Design review of the part built by this model. Coordinates are the model's own, in mm. A direction names the side the tool comes from. Give positions to 0.01 mm unless a question says otherwise; leave off trailing zeros. Write each loop counter-clockwise with the first axis right and the second up, starting at its lowest first coordinate (ties: lowest second). Pieces come first, ordered by that corner, then holes. Notation, with made-up numbers: (-7.5, 32) -> (17.5, 32) arc R24 cw to (17.5, 66) -> close; hole circle Ø7 at (35.25, 50.5). An arc over 180 degrees is marked (long way). Answer as a JSON object with one key per item and string values.
```python
from build123d import *

# Parameters (mm, degrees)
F1_DEPTH = 233
F2_R     = 8.5
F3_DEPTH = 20
F4_R     = 12.5
F5_DEPTH = 15
F7_DEPTH = 15


with BuildPart() as f1:
    # F0 (on Top) → F1 (new body)
    with BuildSketch(Plane.XY):
        Polygon((5, 8.660254), (-5, 8.660254), (-10, 0), (-5, -8.660254), (5, -8.660254), (10, 0), align=None)
    extrude(amount=F1_DEPTH)

    # F2 (on face) → F3 (join)
    with BuildSketch(Plane.XY.offset(233)):
        Circle(F2_R)
    extrude(amount=F3_DEPTH)

    # F4 (on face) → F5 (join)
    with BuildSketch(Plane(origin=(0, 0, 0), x_dir=(1, 0, 0), z_dir=(0, 0, -1))):
        Circle(F4_R)
        Polygon((5, -8.660254), (-5, -8.660254), (-10, 0), (-5, 8.660254), (5, 8.660254), (10, 0), align=None, mode=Mode.SUBTRACT)
        Polygon((-10, 0), (-5, -8.660254), (5, -8.660254), (10, 0), (5, 8.660254), (-5, 8.660254), align=None)
    extrude(amount=F5_DEPTH)

    # F6 (on face) → F7 (join)
    with BuildSketch(Plane(origin=(0, 0, -15), x_dir=(1, 0, 0), z_dir=(0, 0, -1))):
        Polygon((4.953786, -8.686772), (9.999858, -0.053281), (5.046072, 8.633491), (-4.953786, 8.686772), (-9.999858, 0.053281), (-5.046072, -8.633491), align=None)
    extrude(amount=F7_DEPTH)


solid = f1.part
```
(1) For line 1 along Z through (x, y) = (5.5, -8.5); line 2 along Y through (x, z) = (1, 92.5); line 3 along Y through (x, z) = (-0.75, 238), list the stretches that pass through material, from the lowest coordinate up.
Here are the results:
{"line 1": "z = -15 to 0", "line 2": "y = -8.66 to 8.66", "line 3": "y = -8.47 to 8.47"}
(2) For faces 1 (the flat face through (7.535, 4.27, 114.869)), 2 (the flat face through (7.558, -4.229, -22.395)), 3 (the flat face through (0, -8.66, 115)), 4 (the cylindrical face through (4.57, 7.167, 242.86)), 5 (the flat face through (7.44, 4.43, -22.4)), list the 3-axis set-ups (+Z, -Z, +X, -X, +Y, -Y) from which the entire face can be reached by the end or side of a thin tool; tool diameter is ignored.
Here are the results:
{"face 1": "+Z, +X, +Y", "face 2": "-Z, +X, -Y", "face 3": "+Z, +X, -X, -Y", "face 4": "+Z", "face 5": "-Z, +X, +Y"}
(3) We need section B-B, the plane x = 0. State the section outline as (y, z) points, then the cut area to 3 significant figures.
Here are the results:
{"outline": "(-12.5, -15) -> (-8.66, -15) -> (-8.66, -30) -> (8.66, -30) -> (8.66, -15) -> (12.5, -15) -> (12.5, 0) -> (8.66, 0) -> (8.66, 233) -> (8.5, 233) -> (8.5, 253) -> (-8.5, 253) -> (-8.5, 233) -> (-8.66, 233) -> (-8.66, 0) -> (-12.5, 0) -> close", "area": "5,010 mm²"}
(4) Clearance check with flat-ended pins moving along their axes: pin 1 (5 mm diameter, centred on x = -7, z = 218, fed in from -Y); pin 2 (11 mm diameter, centred on x = 2, z = 168.5, fed in from +Y); pin 3 (1 mm diameter, centred on x = 8.5, z = 35, fed in from +Y). State where each tip first meets the part, or that it passes through.
Here are the results:
{"pin 1": "stops at y = -8.66", "pin 2": "stops at y = 8.66", "pin 3": "stops at y = 3.46"}
(5) We need section A-A, the plane z = 199. State the section outline as (x, y) points, then the cut area to 3 significant figures.
Here are the results:
{"outline": "(-10, 0) -> (-5, -8.66) -> (5, -8.66) -> (10, 0) -> (5, 8.66) -> (-5, 8.66) -> close", "area": "260 mm²"}
